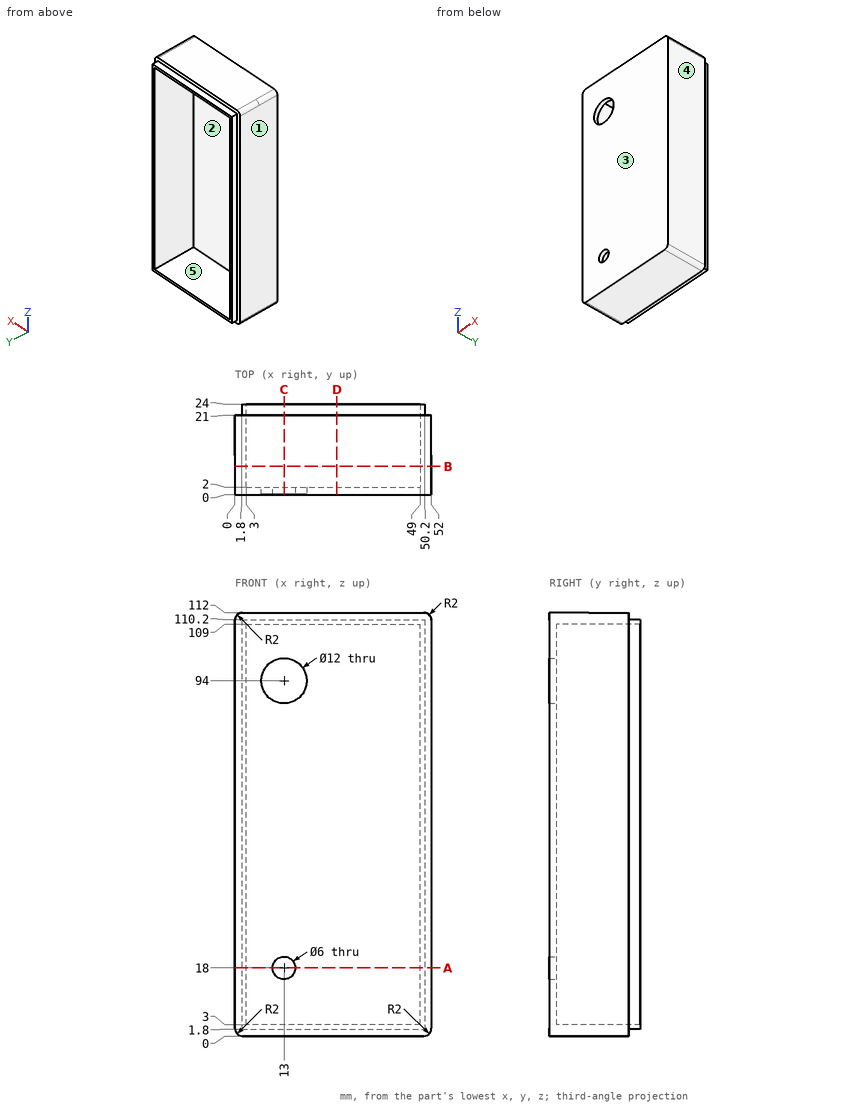
Part print with two shaded views. Sizes in mm from the minimum x, y, z corner. A direction names the side the tool comes from. Coordinates: 2 decimals unless noted, no trailing zeros. Write each loop counter-clockwise with the first axis right and the second up, starting at its lowest first coordinate (ties: lowest second). Pieces come first, ordered by that corner, then holes.
(1) Mould opens along X. For the marked faces 1, 2 and 3 say: pulls with the +X half, pulls with the -X half, needs draft (parallel to the pull), parting line crosses it, or undercut.
(2) Cut at A-A on z = 18. List the corners of the cut face in (x, y), and give its area (3 significant figures).
(3) Cut at C-C on x = 13. List the corners of the cut face in (y, z), and give its area (3 significant figures).
(4) Cut at B-B on y = 7.5. List the corners of the cut face in (x, z).
(5) Cut at D-D on x = 27. List the corners of the cut face in (y, z).
(6) Pin check, flat tips, straight feed: pin 1 Ø1.5 at (y, z) = (23, 34.5) entering from -X; pin 2 Ø2.5 at (x, y) = (35.5, 22.5) entering from +Z; pin 3 Ø12 at (x, z) = (19, 40.5) entering from +Y. Stop position of each tip, or through.
(7) 3-axis set-ups, long thin cutter, end or side, ignore diameter. For the marked faces 4 and 5: which of +Z, -Z, +X, -X, +Y, -Y reach the whole face in a straight line?
(8) Drill centre lines: line 1 (Z direction, x = 28, y = 6.25); line 2 (X direction, y = 14.75, z = 43.5); line 3 (Z direction, x = 13, y = 0.7). Where is each one in solid material? Low to high.
Working result:
1. face 1: pulls with the -X half
1. face 2: undercut
1. face 3: needs draft
2. outline: (0, 0) - (10, 0) - (10, 2) - (3, 2) - (3, 24) - (1.8, 24) - (1.8, 21) - (0, 21) - close; (16, 0) - (52, 0) - (52, 21) - (50.2, 21) - (50.2, 24) - (49, 24) - (49, 2) - (16, 2) - close
2. area: 213 mm2
3. outline: (0, 0) - (21, 0) - (21, 1.8) - (24, 1.8) - (24, 3) - (2, 3) - (2, 15) - (0, 15) - close; (0, 21) - (2, 21) - (2, 88) - (0, 88) - close; (0, 100) - (2, 100) - (2, 109) - (24, 109) - (24, 110.2) - (21, 110.2) - (21, 112) - (0, 112) - close
3. area: 309 mm2
4. outline: (0, 2) arc R2 ccw to (2, 0) - (50, 0) arc R2 ccw to (52, 2) - (52, 110) arc R2 ccw to (50, 112) - (2, 112) arc R2 ccw to (0, 110) - close; hole (3, 3) - (49, 3) - (49, 109) - (3, 109) - close
5. outline: (0, 0) - (21, 0) - (21, 1.8) - (24, 1.8) - (24, 3) - (2, 3) - (2, 109) - (24, 109) - (24, 110.2) - (21, 110.2) - (21, 112) - (0, 112) - close
6. pin 1: stops at x = 1.8
6. pin 2: stops at z = 110.2
6. pin 3: stops at y = 2
7. face 4: +Z, -Z, +X, +Y, -Y
7. face 5: +Y
8. line 1: z = 0 to 3, 109 to 112
8. line 2: x = 0 to 3, 49 to 52
8. line 3: z = 0 to 15, 21 to 88, 100 to 112
